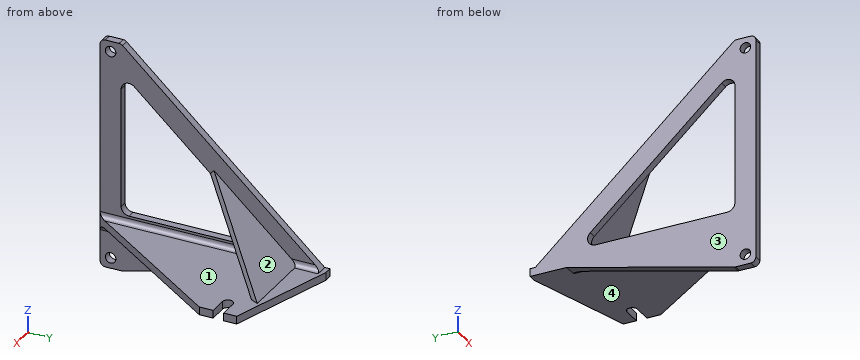
from build123d import *

# Parameters (mm, degrees)
SKETCH_1_R          = 2
EXTRUDE_1_DEPTH     = 3
SKETCH_2_W          = 3
SKETCH_2_H          = 86
EXTRUDE_2_DEPTH     = 44
CUT_EXTRUDE_1_DEPTH = 3
FILLET_1_R          = 2
RIB_2_REACH         = 105.226
SKETCH_8_WALL_W     = 259.89004629
SKETCH_8_WALL_H     = 2
FILLET_2_R          = 2


with BuildPart() as part:
    # Sketch 1 → Extrude 1 (new body)
    with BuildSketch(Plane(origin=(0, 0, 0), x_dir=(0, 0, -1), z_dir=(1, 0, 0))):
        Polygon((-44, 0), (44, 0), (44, 8), (25, 84.048968678), (-44, 8), align=None)
        with Locations((-40, 4)):
            Circle(SKETCH_1_R, mode=Mode.SUBTRACT)
        with Locations(Location((40, 4, 0), (0, 0, 180))):
            Circle(SKETCH_1_R, mode=Mode.SUBTRACT)
        with BuildLine():
            Line((-28.646958906, 13.01585119), (16.806444582, 63.112727395))
            ThreePointArc((16.806444582, 63.112727395), (20.10865764, 63.895569238), (22.028233046, 61.096876205))
            Line((22.028233046, 61.096876205), (22.028233046, 11))
            ThreePointArc((22.028233046, 11), (21.14955339, 8.878679656), (19.028233046, 8))
            Line((19.028233046, 8), (-26.425170442, 8))
            ThreePointArc((-26.425170442, 8), (-29.168120821, 9.785000735), (-28.646958906, 13.01585119))
        make_face(mode=Mode.SUBTRACT)
    extrude(amount=EXTRUDE_1_DEPTH)

    # Sketch 2 → Extrude 2 (add)
    with BuildSketch(Plane(origin=(0, 0, 0), x_dir=(0, 0, -1), z_dir=(1, 0, 0))):
        with Locations((26.5, 43)):
            Rectangle(SKETCH_2_W, SKETCH_2_H)
    extrude(amount=EXTRUDE_2_DEPTH)

    # Sketch 3 → Cut-Extrude 1 (cut)
    with BuildSketch(Plane.XY.offset(-25)):
        with BuildLine():
            Line((3, 86), (44, 73))
            Line((44, 73), (44, 68))
            Line((44, 68), (37, 68))
            ThreePointArc((37, 68), (35, 66), (37, 64))
            Line((37, 64), (44, 64))
            Line((44, 64), (47.670015823, 64))
            Line((47.670015823, 64), (3, 0))
            Line((3, 0), (48.684950213, 0))
            Line((48.684950213, 0), (53.414147697, 0))
            Line((53.414147697, 0), (53.414147697, 86))
            Line((53.414147697, 86), (3, 86))
        make_face()
    extrude(amount=-CUT_EXTRUDE_1_DEPTH, mode=Mode.SUBTRACT)

    # Fillet 1
    fillet_1_edges = [part.edges().sort_by_distance(p)[0] for p in [
        (3, 36.020618391, -28),
        (3, 42.024484339, -25),
    ]]
    fillet(fillet_1_edges, radius=FILLET_1_R)

    # Sketch 8 wall → Rib 2 (add, up to next)
    with BuildSketch(Plane(origin=(17.70715676, 57.665222316, -11.863868016), x_dir=(0.571832945578, 0.60756293308, -0.551248006526), z_dir=(0.82037008865, -0.42349728062, 0.384243374641)), mode=Mode.PRIVATE) as rib_2_sk1:
        with Locations((0, 1)):
            Rectangle(SKETCH_8_WALL_W, SKETCH_8_WALL_H)
    rib_2_tool1 = extrude(rib_2_sk1.sketch, amount=-RIB_2_REACH, mode=Mode.PRIVATE) - part.part
    add(rib_2_tool1.solids().sort_by_distance((17.70715676, 57.665222316, -11.863868016))[0])

    # Fillet 2
    fillet_2_edges = [part.edges().sort_by_distance(p)[0] for p in [
        (1.5, 8, 44),
        (1.5, 8, -44),
        (1.5, 0, -44),
        (1.5, 0, 44),
    ]]
    fillet(fillet_2_edges, radius=FILLET_2_R)


solid = part.part
Verification items for the finished model (mm, model axes). Face numbers are marked on the shaded views. Give positions to 0.01 mm unless a question says otherwise; leave off trailing zeros. Write each loop counter-clockwise with the first axis right and the second up, starting at its lowest first coordinate (ties: lowest second). Pieces come first, ordered by that corner, then holes.
(1) Cross-section at D-D (z = 14.5). Enter the section's corners in (x, y).
(2) Gauge pin test, flat ends, axial feed: pin 1 (13 mm diameter, centred on x = 15.5, y = 33.5, fed in from -Z); pin 2 (2.5 mm diameter, centred on y = 4, z = 40, fed in from -X); pin 3 (2.5 mm diameter, centred on x = 1, z = -5, fed in from +Y); pin 4 (2 mm diameter, centred on y = 13, z = -28, fed in from -X). Record the tip position at first contact, or that the pin passes through.
(3) Cross-section at B-B (y = 38). Enter the section's corners in (x, z), plus the area to 3 significant figures.
(4) Mould release check, pull along Z, two halves, no side actions. Record for the marked faces 1, 2, 3 and 4: +Z half, -Z half, draft (parallel to the pull), parting line (faces both ways), or undercut.
(5) Cross-section at C-C (x = 20). Enter the section's corners in (y, z).
(6) Cross-section at A-A (z = -8). Enter the section's corners in (x, y), plus the area to 3 significant figures.
(7) Material ranges on line 1 (X direction, y = 24, z = -33); line 2 (Z direction, x = 19.5, y = 63); line 3 (Z direction, x = 18.5, y = 67), recorded low to high.
Worked out:
1. outline: (0, 0) - (3, 0) - (3, 8) - (0, 8) - close; (0, 28.61) - (3, 28.61) - (3, 40.51) - (0, 40.51) - close
2. pin 1: stops at z = -28
2. pin 2: passes through
2. pin 3: stops at y = 63.38
2. pin 4: stops at x = 0
3. outline: (0, -36.5) - (3, -36.5) - (3, -30) arc R2 cw to (5, -28) - (29.52, -28) - (29.52, -25) - (5, -25) arc R2 cw to (3, -23) - (3, -22.03) - (0, -22.03) - close; (0, 5.98) - (3, 5.98) - (3, 16.78) - (0, 16.78) - close
3. area: 157 mm2
4. face 1: undercut
4. face 2: +Z half
4. face 3: draft
4. face 4: -Z half
5. outline: (24.36, -28) - (80.61, -28) - (80.61, -25) - (75.12, -25) - (61.45, -12.59) - (60.1, -14.07) - (72.14, -25) - (24.36, -25) - close
6. outline: (0, 0) - (3, 0) - (3, 8) - (0, 8) - close; (0, 53.41) - (13.7, 53.41) - (15.24, 56.38) - (3, 56.38) - (3, 65.31) - (0, 65.31) - close
6. area: 93.8 mm2
7. line 1: x = 0 to 3
7. line 2: z = -28 to -25, -16.7 to -14
7. line 3: z = -28 to -25, -20.33 to -17.63
